from build123d import *

# Parameters (mm, degrees)
F0_R     = 0.75
F0_R_2   = 0.53
F1_DEPTH = 1


# Not quite as in the source:
# - a feature names something its author has since deleted; it is built from what else it names


with BuildPart() as f1:
    # F0 (on Right) → F1 (new body)
    with BuildSketch(Plane.YZ):
        Polygon((8.384144865, 0), (0, 0), (0, -11.5), (11.5, -11.5), (11.5, 0), (10.384144865, 0), align=None)
        with Locations((1.7500000088, -9.75)):
            Circle(F0_R, mode=Mode.SUBTRACT)
        with Locations((1.75, -7.75)):
            Circle(F0_R, mode=Mode.SUBTRACT)
        with Locations((3.7499851588, -10.5567658602)):
            Circle(F0_R_2, mode=Mode.SUBTRACT)
        with Locations((5.7499653617, -9.750009894)):
            Circle(F0_R, mode=Mode.SUBTRACT)
        with Locations((3.7499885936, -8.7499999912)):
            Circle(F0_R, mode=Mode.SUBTRACT)
        with Locations((3.7499923957, -6.75)):
            Circle(F0_R, mode=Mode.SUBTRACT)
        with Locations((5.7499752647, -7.7500098941)):
            Circle(F0_R, mode=Mode.SUBTRACT)
        with Locations((1.75, -5.75)):
            Circle(F0_R, mode=Mode.SUBTRACT)
        with Locations((1.75, -3.75)):
            Circle(F0_R, mode=Mode.SUBTRACT)
        with Locations((1.75, -1.75)):
            Circle(F0_R, mode=Mode.SUBTRACT)
        with Locations((3.7499961979, -4.75)):
            Circle(F0_R, mode=Mode.SUBTRACT)
        with Locations((5.7499851588, -5.7500098941)):
            Circle(F0_R, mode=Mode.SUBTRACT)
        with Locations((5.7499950529, -3.7500098941)):
            Circle(F0_R, mode=Mode.SUBTRACT)
        with Locations((3.75, -2.75)):
            Circle(F0_R, mode=Mode.SUBTRACT)
        with Locations((3.75, -0.94325)):
            Circle(F0_R_2, mode=Mode.SUBTRACT)
        with Locations((7.749955461, -10.5567658602)):
            Circle(F0_R_2, mode=Mode.SUBTRACT)
        with Locations((7.7499520262, -8.7500197836)):
            Circle(F0_R, mode=Mode.SUBTRACT)
        with Locations((7.7499680167, -6.7500197925)):
            Circle(F0_R, mode=Mode.SUBTRACT)
        with Locations((9.7499307145, -9.750039585)):
            Circle(F0_R, mode=Mode.SUBTRACT)
        with Locations((9.749950516, -7.7500395851)):
            Circle(F0_R, mode=Mode.SUBTRACT)
        with Locations((7.7499840072, -4.7500197926)):
            Circle(F0_R, mode=Mode.SUBTRACT)
        with Locations((5.750004947, -1.7500098941)):
            Circle(F0_R, mode=Mode.SUBTRACT)
        with Locations((7.7499999977, -2.7500197927)):
            Circle(F0_R, mode=Mode.SUBTRACT)
        with Locations((7.7499999977, -0.9432697927)):
            Circle(F0_R_2, mode=Mode.SUBTRACT)
        with Locations((9.7499703087, -5.7500395852)):
            Circle(F0_R, mode=Mode.SUBTRACT)
        with Locations((9.7499901013, -3.7500395853)):
            Circle(F0_R, mode=Mode.SUBTRACT)
        with Locations((9.750009894, -1.7500395854)):
            Circle(F0_R, mode=Mode.SUBTRACT)
    extrude(amount=F1_DEPTH)


solid = f1.part
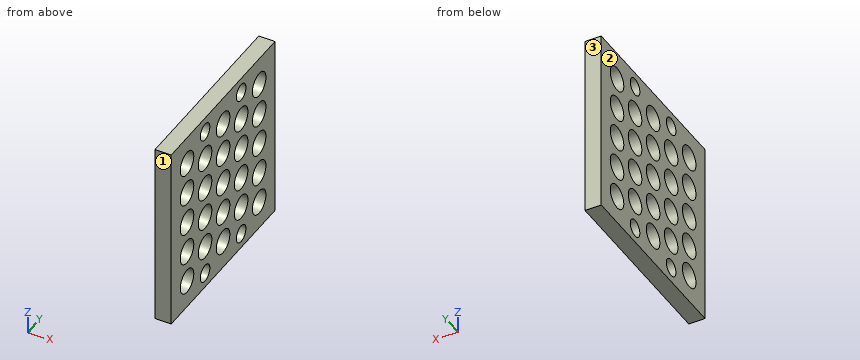
Geometry check sheet. Reference: the model listing, model coordinates, mm. Face numbers are marked on the shaded views. Round coordinates to 2 decimals unless told otherwise and drop trailing zeros. Order: outer loops, then holes, each group sorted by start corner. A loop starts at its lowest first (then second) coordinate and runs counter-clockwise, first axis right, second up. Notation, with made-up numbers: M -8,-40 L 7,-40 A31 ccw 7,-15 Z; hole C 17,23 d8. An arc over 180 degrees is marked long. Answer in a Markdown table with one row per item. Add a question column.
Item 1: Sectioned sample at A-A, the plane y = 3.75. Enter the section's corners in (x, z).
Item 2: Sectioned sample at C-C, the plane x = 0.65. State how many separate pieces and enclosed holes the cut face has, plus the area to 3 significant figures.
Item 3: Draft check along Y on the marked faces 1, 2 and 3. Enter one of: released by +Y, released by -Y, zero draft, split by the parting line, or undercut.
Item 4: Sectioned sample at B-B, the plane y = 5.75. Enter the section's corners in (x, z).
Item 5: Sectioned sample at D-D, the plane y = 9.5. Enter the section's corners in (x, z).
Item 6: Depth check by flat-ended pin: pin 1 Ø1.2 at (y, z) = (5.75, -9.75) entering from +X. Enter the tip coordinate at first touch or a pass-through.
Item 7: Material ranges on L1, parallel to Z at x = 0.6, y = 1.75; L2, parallel to Y at x = 0.2, z = -0.5; L3, parallel to Y at x = 0.2, z = -2.25, recorded low to high. Write a range as [from, to].
Filled in:
| question | item | result |
|---|---|---|
| 1 | outline | M 0,-11.5 L 1,-11.5 L 1,-11.09 L 0,-11.09 Z; M 0,-10.03 L 1,-10.03 L 1,-9.5 L 0,-9.5 Z; M 0,-8 L 1,-8 L 1,-7.5 L 0,-7.5 Z; M 0,-6 L 1,-6 L 1,-5.5 L 0,-5.5 Z; M 0,-4 L 1,-4 L 1,-3.5 L 0,-3.5 Z; M 0,-2 L 1,-2 L 1,-1.47 L 0,-1.47 Z; M 0,-0.41 L 1,-0.41 L 1,0 L 0,0 Z |
| 2 | separate pieces | 1 |
| 2 | enclosed holes | 27 |
| 2 | area | 88.1 mm² |
| 3 | face 1 | released by -Y |
| 3 | face 2 | zero draft |
| 3 | face 3 | released by +Y |
| 4 | outline | M 0,-11.5 L 1,-11.5 L 1,-10.5 L 0,-10.5 Z; M 0,-9 L 1,-9 L 1,-8.5 L 0,-8.5 Z; M 0,-7 L 1,-7 L 1,-6.5 L 0,-6.5 Z; M 0,-5 L 1,-5 L 1,-4.5 L 0,-4.5 Z; M 0,-3 L 1,-3 L 1,-2.5 L 0,-2.5 Z; M 0,-1 L 1,-1 L 1,0 L 0,0 Z |
| 5 | outline | M 0,-11.5 L 1,-11.5 L 1,-10.46 L 0,-10.46 Z; M 0,-9.04 L 1,-9.04 L 1,-8.46 L 0,-8.46 Z; M 0,-7.04 L 1,-7.04 L 1,-6.46 L 0,-6.46 Z; M 0,-5.04 L 1,-5.04 L 1,-4.46 L 0,-4.46 Z; M 0,-3.04 L 1,-3.04 L 1,-2.46 L 0,-2.46 Z; M 0,-1.04 L 1,-1.04 L 1,0 L 0,0 Z |
| 6 | pin 1 | passes through |
| 7 | L1 | z = [-11.5, -10.5], [-9, -8.5], [-7, -6.5], [-5, -4.5], [-3, -2.5], [-1, 0] |
| 7 | L2 | y = [0, 3.46], [4.04, 7.46], [8.04, 11.5] |
| 7 | L3 | y = [0, 1.19], [2.31, 3.19], [4.31, 5.19], [6.31, 7.19], [8.31, 9.19], [10.31, 11.5] |
